```python
from build123d import *

# Parameters (mm, degrees)
F0_W     = 38.1
F0_H     = 63.5
F1_DEPTH = 25.4
F2_W     = 19.05
F2_H     = 26.9875
F3_DEPTH = 25.4
F4_R     = 6.35
F5_DEPTH = 25.4
F6_DEPTH = 3.175
F7_SIZE  = 6.35


with BuildPart() as f1:
    # F0 (on Top) → F1 (new body)
    with BuildSketch(Plane.XY):
        Rectangle(F0_W, F0_H)
    extrude(amount=F1_DEPTH)

    # F2 (on face) → F3 (cut)
    with BuildSketch(Plane.XY.offset(25.4)):
        with Locations((-9.525, -18.25625)):
            Rectangle(F2_W, F2_H)
    extrude(amount=-F3_DEPTH, mode=Mode.SUBTRACT)

    # F4 (on face) → F5 (cut)
    with BuildSketch(Plane.YZ.offset(19.05)):
        with Locations((-19.05, 12.7)):
            Circle(F4_R)
    extrude(amount=-F5_DEPTH, mode=Mode.SUBTRACT)

    # F6 (cut): a face of the model
    f6_faces = [f1.faces().sort_by_distance(p)[0] for p in [
        (-9.525, -4.7625, 12.7),
    ]]
    extrude(f6_faces, amount=-F6_DEPTH, mode=Mode.SUBTRACT)

    # F7
    f7_edges = [f1.edges().sort_by_distance(p)[0] for p in [
        (-9.525, -1.5875, 25.4),
        (-9.525, -1.5875, 0),
    ]]
    chamfer(f7_edges, length=F7_SIZE)


solid = f1.part
```
CAD build for the part. Positions are in the model's coordinates, mm. A direction names the side the tool comes from. Round coordinates to 2 decimals unless told otherwise and drop trailing zeros. Loops run counter-clockwise (first coordinate to the right, second up) from the corner with the lowest first, then second, coordinate; pieces in that order, holes last. Notation, with made-up numbers: M -9.75,9 L 38.25,9 A22 ccw 38.25,21 Z; hole C 60,32 d11. An arc over 180 degrees is marked long. Use a Markdown table: item, result. Add a question column.
(1) Cut at C-C (x = 16.5). Give the cut face in (y, z), and give its area (3 significant figures).
(2) Drill centre lines: line 1 (Z direction, x = 4.75, y = -19.05); line 2 (X direction, y = -3, z = 10); line 3 (Y direction, x = 8, z = 10.5). Where is each one in solid material? Low to high.
(3) Flat gauge pin, fed straight in: pin 1 (6.5 mm diameter, centred on x = -14, z = 11, fed in from -Y). Where does the tip first touch, or does it go through?
(4) Cut at A-A (z = 12.7). Give the cut face in (x, y), and give its area (3 significant figures).
(5) Cut at D-D (x = -16). Give the cut face in (y, z), and give its area (3 significant figures).
(6) Pull direction Z, two halves, no side cores. Call faces 1 (the face through (9.658, -19.877, 18.996)), 2 (the face through (-9.66, 1.63, 22.27)), 3 (the face through (4, 8, 0)), 4 (the face through (9, -31.75, 13)): +Z half, -Z half, draft (parallel to the pull), parting line (faces both ways), or undercut.
(7) Cut at B-B (y = -19.05). Give the cut face in (x, z).
(8) Which spindle directions (+Z, -Z, +X, -X, +Y, -Y) get a long thin tool onto all of the face, cutting with end or side? Do faces 5 (the face through (-19.05, 15, 13)), 6 (the face through (-10, -1.588, 13)), 7 (the face through (-9.66, 1.63, 3.13)). Say none if no direction does.
Geometry says:
| question | item | result |
|---|---|---|
| 1 | outline | M -31.75,0 L 31.75,0 L 31.75,25.4 L -31.75,25.4 Z; hole C -19.05,12.7 d12.7 |
| 1 | area | 1,490 mm² |
| 2 | line 1 | z = 0 to 6.35, 19.05 to 25.4 |
| 2 | line 2 | x = 0 to 19.05 |
| 2 | line 3 | y = -31.75 to -25.01, -13.09 to 31.75 |
| 3 | pin 1 | stops at y = -1.59 |
| 4 | outline | M -19.05,-1.59 L 0,-1.59 L 0,-12.7 L 19.05,-12.7 L 19.05,31.75 L -19.05,31.75 Z; M 0,-31.75 L 19.05,-31.75 L 19.05,-25.4 L 0,-25.4 Z |
| 4 | area | 1,600 mm² |
| 5 | outline | M -1.59,6.35 L 4.76,0 L 31.75,0 L 31.75,25.4 L 4.76,25.4 L -1.59,19.05 Z |
| 5 | area | 806 mm² |
| 6 | face 1 | undercut |
| 6 | face 2 | +Z half |
| 6 | face 3 | -Z half |
| 6 | face 4 | draft |
| 7 | outline | M 0,0 L 19.05,0 L 19.05,6.35 L 0,6.35 Z; M 0,19.05 L 19.05,19.05 L 19.05,25.4 L 0,25.4 Z |
| 8 | face 5 | +Z, -Z, -X, +Y, -Y |
| 8 | face 6 | +Z, -Z, -X, -Y |
| 8 | face 7 | -Z, -X, -Y |
